Geometry: see drawing. Coordinates: mm, zero at the bounding-box minimum. A direction names the side the tool comes from. Coordinates: 2 decimals unless noted, no trailing zeros. Write each loop counter-clockwise with the first axis right and the second up, starting at its lowest first coordinate (ties: lowest second). Pieces come first, ordered by that corner, then holes. Notation, with made-up numbers: (-11, -26) - (37, -26) arc R5 ccw to (37, -20) - close; hole circle Ø2 at (33.5, 57.5). An arc over 180 degrees is marked (long way). Use CSV: the item, a comma, the result in double quotes.
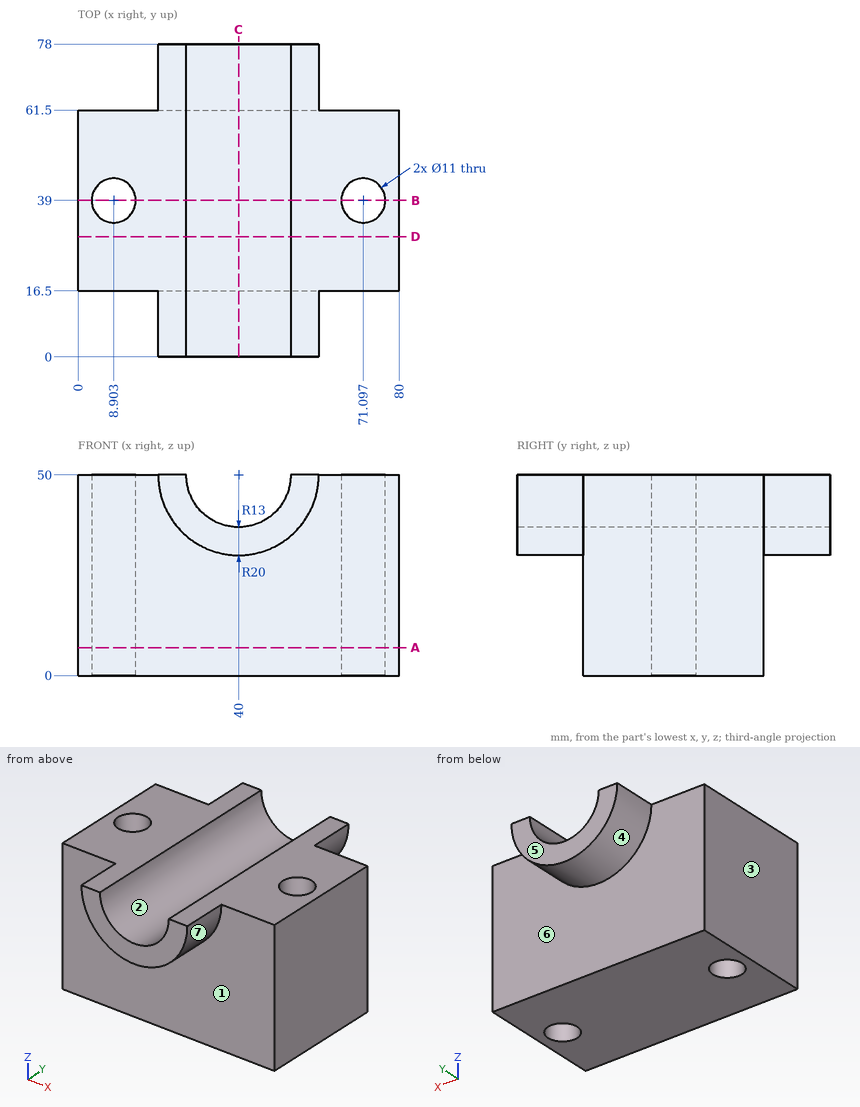
(1) Draft query along X for the marked faces 1, 2, 3 and 4. Return one class per face: pulls with the +X half, pulls with the -X half, needs draft (parallel to the pull), parting line crosses it, or undercut.
Check values:
face 1,"needs draft"
face 2,"undercut"
face 3,"pulls with the -X half"
face 4,"parting line crosses it"
(2) Cut plane D-D on y = 30. Return loops of the section in (x, z).
Check values:
outline,"(0, 0) - (80, 0) - (80, 50) - (53, 50) arc R13 cw to (27, 50) - (0, 50) - close"
(3) Cut plane C-C on x = 40. Return loops of the section in (y, z).
Check values:
outline,"(0, 30) - (16.5, 30) - (16.5, 0) - (61.5, 0) - (61.5, 30) - (78, 30) - (78, 37) - (0, 37) - close"
(4) Cut plane B-B on y = 39. Return loops of the section in (x, z).
Check values:
outline,"(0, 0) - (3.4, 0) - (3.4, 50) - (0, 50) - close; (14.4, 0) - (65.6, 0) - (65.6, 50) - (53, 50) arc R13 cw to (27, 50) - (14.4, 50) - close; (76.6, 0) - (80, 0) - (80, 50) - (76.6, 50) - close"
(5) Ray query, probe 1 along Y at (x, z) = (71, 14.5); probe 2 along X at (y, z) = (40.5, 17) (1 decimal); probe 3 along Y at (x, z) = (42, 18). Return the intervals inside material, ascending. Write a range as from..to.
Check values:
probe 1,"16.5..33.5, 44.5..61.5"
probe 2,"0..3.6, 14.2..65.8, 76.4..80"
probe 3,"16.5..61.5"
(6) Reachability of the marked faces 5, 6 and 7 from +Z, -Z, +X, -X, +Y, -Y: full face, straight path, thin tool, end or side. Return the list, or none.
Check values:
face 5,"+Z, -Z, +X, -X, +Y"
face 6,"-Z, +Y"
face 7,"-Z, -Y"
(7) Cut plane A-A on z = 7. Return loops of the section in (x, y).
Check values:
outline,"(0, 16.5) - (80, 16.5) - (80, 61.5) - (0, 61.5) - close; hole circle Ø11 at (8.9, 39); hole circle Ø11 at (71.1, 39)"
(8) Pin query (flat end, axial travel): pin 1 Ø6 at (x, y) = (31, 63.5) entering from +Z; pin 2 Ø10 at (x, z) = (66.5, 44) entering from +Y; pin 3 Ø1.5 at (x, y) = (31, 66) entering from +Z; pin 4 Ø9 at (x, y) = (8.9, 39) entering from -Z. Return the tip coordinate at first contact, or that it passes through.
Check values:
pin 1,"z = 45"
pin 2,"y = 61.5"
pin 3,"z = 41.4"
pin 4,"through"
